Autodesk Inventor part; units mm, degrees
ref_plane "Work Plane1" through (0, 2, 0) normal (0, -1, 0) x (1, 0, 0)
ref_plane "YZ Plane" through (0, 0, 0) normal (1, 0, 0) x (0, 1, 0)
ref_plane "XZ Plane" through (0, 0, 0) normal (0, 1, 0) x (-1, 0, 0)
sketch "Sketch1" plane through (0, 0, 0) normal (0, 0, 1) x (1, 0, 0)
  line L0 (0, 0) -> (3, 0)
  line L1 (3, 0) -> (3, 10)
  line L2 (3, 10) -> (13, 10)
  line L3 (13, 10) -> (13, -3)
  line L4 (13, -3) -> (0, -3)
  line L5 (0, -3) -> (0, 0)
  dimension "d0" = 10
  dimension "d1" = 3
  dimension "d2" = 3
  dimension "d3" = 10
extrude "Extrusion1" add sketch "Sketch1" along normal blind 33
sketch "Sketch2" plane through (0, -3, 0) normal (0, -1, 0) x (1, 0, 0)
  line L0 (13, 0) -> (3, 0)
  line L1 (3, 0) -> (3, 33)
  line L2 (13, 33) -> (3, 33)
  line L3 (13, 0) -> (13, 33)
  line L4 (0, 33) -> (13, 33)
  line L5 (6.3546, 24.45) -> (4.7091, 27.3)
  line L6 (4.7091, 27.3) -> (6.3546, 30.15)
  line L7 (6.3546, 30.15) -> (9.6454, 30.15)
  line L8 (9.6454, 30.15) -> (11.2909, 27.3) construction
  line L9 (11.2909, 27.3) -> (9.6454, 24.45) construction
  line L10 (9.6454, 24.45) -> (6.3546, 24.45)
  line L11 (6.3546, 2.85) -> (4.7091, 5.7)
  line L12 (4.7091, 5.7) -> (6.3546, 8.55)
  line L13 (6.3546, 8.55) -> (9.6454, 8.55)
  line L14 (9.6454, 8.55) -> (11.2909, 5.7) construction
  line L15 (11.2909, 5.7) -> (9.6454, 2.85) construction
  line L16 (9.6454, 2.85) -> (6.3546, 2.85)
  line L17 (9.6454, 30.15) -> (9.6454, 24.45) construction
  line L18 (9.6454, 24.45) -> (13, 24.45)
  line L19 (13, 24.45) -> (13, 30.15)
  line L20 (13, 30.15) -> (9.6454, 30.15)
  line L21 (9.6454, 8.55) -> (9.6454, 2.85) construction
  line L22 (9.6454, 2.85) -> (13, 2.85)
  line L23 (13, 2.85) -> (13, 8.55)
  line L24 (13, 8.55) -> (9.6454, 8.55)
  line L25 (13, 0) -> (13, 33)
  point P0 (0, 0)
  point P1 (8, 27.3)
  point P2 (8, 5.7)
  point P3 (8, 33)
  point P4 (6.5, 33)
  point P5 (8, 27.3)
  point P6 (8, 5.7)
  point P7 (13, 8.55)
  point P8 (13, 30.15)
  dimension "d6" = 21.6
  dimension "d7" = 5.7
  dimension "d8" = 5.7
  dimension "d19" = 5.7
hole "Hole1" at (8, -3, 27.3) at (8, -3, 5.7) direction (0, 1, 0) diameter 3.2 end through all countersink diameter 6 countersink angle 90
sketch "Sketch3" plane through (0, -3, 0) normal (0, -1, 0) x (1, 0, 0)
  circle A0 centre (8, 27.3) radius 3
  circle A1 centre (8, 5.7) radius 3
  line L0 (0, 0) -> (13, 0)
  line L1 (13, 0) -> (13, 33)
  line L2 (0, 33) -> (13, 33)
  line L3 (0, 0) -> (0, 33)
  circle A2 centre (8, 5.7) radius 3
  circle A3 centre (8, 5.7) radius 1.6
  circle A4 centre (8, 27.3) radius 3
  circle A5 centre (8, 27.3) radius 1.6
  line L4 (13, 28) -> (8, 28)
  line L5 (8, 28) -> (8, 26.6)
  line L6 (8, 26.6) -> (13, 26.6)
  line L7 (13, 26.6) -> (13, 28)
  line L8 (13, 6.4) -> (8, 6.4)
  line L9 (8, 6.4) -> (8, 5)
  line L10 (8, 5) -> (13, 5)
  line L11 (13, 5) -> (13, 6.4)
  point P0 (0, 0)
  point P1 (13, 16.5)
  dimension "d16" = 1.4
extrude "Extrusion2" cut sketch "Sketch3" against normal blind 1.4 contours A0 L6 A5 L4 | A0 L4 L1 L6 | A5 L6 L5 L4 | L1 L10 A1 L8 | A1 L10 A3 L8 | A3 L10 L9 L8 picked at (10.0575, 27.1414) picked at (8.5333, 27.3) picked at (10.0575, 5.8586) picked at (8.5333, 5.7)
ref_plane "Work Plane1" through (0, 2, 0) normal (0, -1, 0) x (1, 0, 0)
extrude "Extrusion3" cut sketch "Sketch2" against normal blind 3 from surface at -5 contours L22 L16 L11 L12 L13 L24 L3 | L18 L10 L5 L6 L7 L20 L3
sketch "Sketch4" plane through (13, -3, 0) normal (1, 0, 0) x (0, 0, -1)
  line L0 (0, 13) -> (-33, 13)
  line L1 (-16.5, 13) -> (-16.5, 0)
  line L2 (-6.4, 0) -> (-26.6, 0)
  line L3 (-14.5, 11) -> (-13, 11)
  line L4 (-13, 11) -> (-13, 8)
  line L5 (-13, 8) -> (-14.5, 8)
  line L6 (-14.5, 8) -> (-14.5, 11)
  point P0 (0, 3)
  dimension "d23" = 3
  dimension "d24" = 1.5
  dimension "d25" = 2
  dimension "d26" = 2
revolve "Revolution1" cut sketch "Sketch4" angle 360 about axis through (13, 10, 16.5) along (0, -1, 0)
properties part number "hotend magnet"
Geometry: final body of the model. Coordinates: model frame, mm. A direction names the side the tool comes from. Round coordinates to 2 decimals unless told otherwise and drop trailing zeros. Order: outer loops, then holes, each group sorted by start corner. A loop starts at its lowest first (then second) coordinate and runs counter-clockwise, first axis right, second up. Notation, with made-up numbers: M 64.25,-38 L 117.25,-38 A16 cw 117.25,-24 Z; hole C 5.5,3 d4. An arc over 180 degrees is marked long. Use one line per item in the form item = value. Start each with the question number.
Q1. Cut plane A-A (x = 8). Count the separate pieces of the cut face and the enclosed holes in it, and give its area (3 significant figures).
Q2. Access query for faces 4 (the face through (12, -2, 28)), 5 (the face through (1, 0, 16)), 6 (the face through (10, 3, 8.55)), 7 (the face through (10, 5, 17)). Directions: +Z, -Z, +X, -X, +Y, -Y. A direction counts if a zero-diameter tool reaches every point of the face in a straight line with its end or side. Return the directions, or none.
Q3. Mould query, pull axis Z, two halves, no side actions, for faces 1 (the face through (8, 4, 33)), 2 (the face through (3, 5, 16)), 3 (the face through (12, -2, 6.4)). Classes: +Z half, -Z half, draft (parallel to the pull), parting line (faces both ways), or undercut.
Q4. Pin query (flat end, axial travel): pin 1 Ø3 at (y, z) = (8, 15.5) entering from -X; pin 2 Ø3.5 at (x, z) = (8, 5.7) entering from -Y. Return the tip coordinate at first contact, or that it passes through.
Q5. Cut plane C-C (z = 16.5). Return loops of the section in (x, y).
Q6. Cut plane D-D (x = 12.25). Return loops of the section in (y, z).
Q7. Cut plane B-B (y = 6.75). Return loops of the section in (x, z), and give its area (3 significant figures).
Q8. Material intervals for line 1 (Z direction, x = 8, y = 8.6); line 2 (X direction, y = 0.2, z = 27.3); line 3 (Z direction, x = 9, y = 0.5), sorted ascending. Write a range as [from, to].
Geometry results:
q1.separate_pieces = 3
q1.enclosed_holes = 0
q1.area = 327 mm^2
q2.face_4 = +X, -Y
q2.face_5 = +Z, -Z, -X, +Y
q2.face_6 = +X
q2.face_7 = none
q3.face_1 = +Z half
q3.face_2 = draft
q3.face_3 = undercut
q4.pin_1 = 3
q4.pin_2 = -1.75
q5.outline = M 0,-3 L 13,-3 L 13,10 L 3,10 L 3,0 L 0,0 Z; hole M 9.5,5 L 11,5 L 11,8 L 9.5,8 Z
q6.outline = M -3,0 L 10,0 L 10,33 L -3,33 L -3,28 L -1.6,28 L -1.6,26.6 L -3,26.6 L -3,6.4 L -1.6,6.4 L -1.6,5 L -3,5 Z; hole M 2,2.85 L 5,2.85 L 5,8.55 L 2,8.55 Z; hole M 2,24.45 L 5,24.45 L 5,30.15 L 2,30.15 Z; hole M 5,13.08 L 8,13.08 L 8,14.65 L 5,14.65 Z; hole M 5,18.35 L 8,18.35 L 8,19.92 L 5,19.92 Z
q7.outline = M 3,0 L 13,0 L 13,13 A3.5 cw 13,20 L 13,33 L 3,33 Z; M 13,14.5 L 13,18.5 A2 ccw Z; hole C 8,5.7 d3.2; hole C 8,27.3 d3.2
q7.area = 301 mm^2
q8.line_1 = [0, 4.1], [7.3, 25.7], [28.9, 33]
q8.line_2 = [3, 6.4], [9.6, 13]
q8.line_3 = [0, 4.45], [6.95, 26.05], [28.55, 33]
